Geometry check sheet. Reference: drawing and pictorial views, mm from the part's lowest x, y, z. Coordinates: 2 decimals unless noted, no trailing zeros. Write each loop counter-clockwise with the first axis right and the second up, starting at its lowest first coordinate (ties: lowest second). Pieces come first, ordered by that corner, then holes. Notation, with made-up numbers: (16, -30.5) -> (68, -30.5) arc R32 ccw to (68, 6.5) -> close; hole circle Ø11 at (89.25, -22.75). An arc over 180 degrees is marked (long way). Use a Markdown table: item, result.
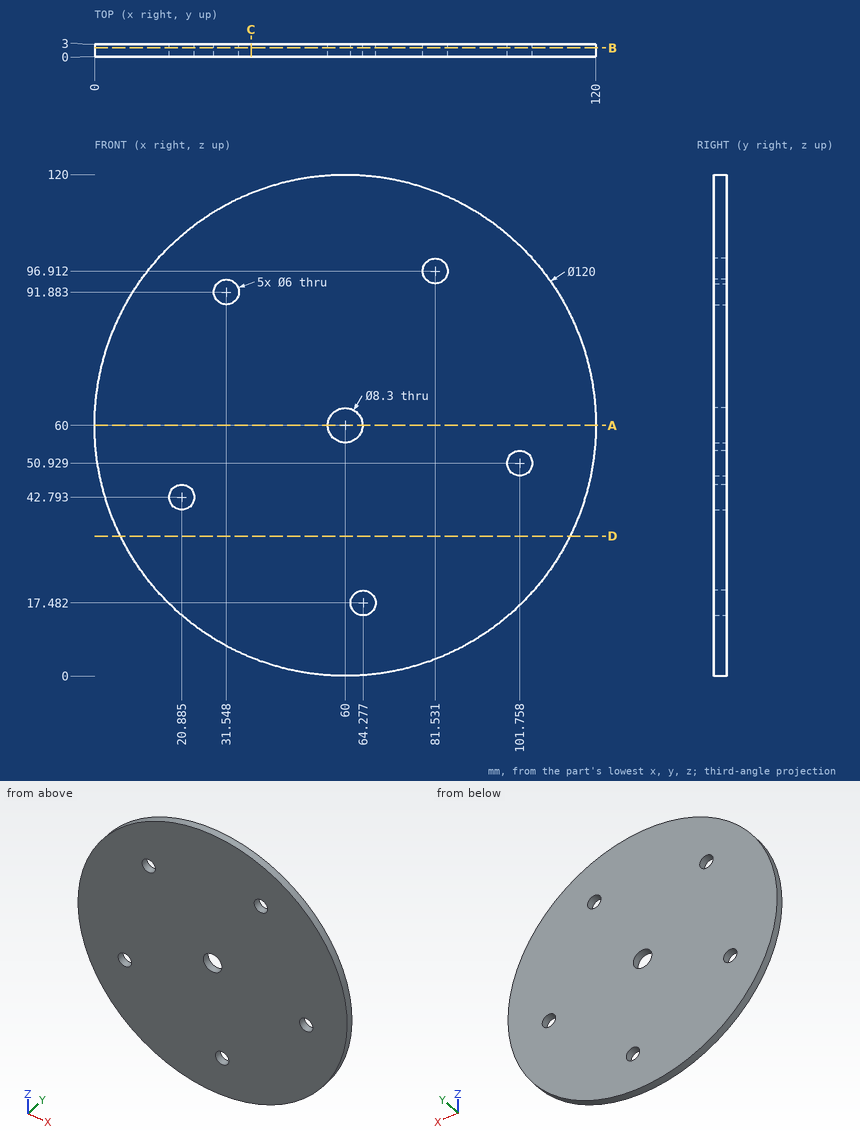
Item 1: Section check D-D on z = 33.5. Record the boundary of the cut face in (x, y), then the cut area to 3 significant figures.
Answer block:
| item | result |
|---|---|
| outline | (6.17, 0) -> (113.83, 0) -> (113.83, 3) -> (6.17, 3) -> close |
| area | 323 mm^2 |
Item 2: Section check B-B on y = 2.1. Count the separate pieces of the cut face and the enclosed holes in it, then the cut area to 3 significant figures.
Answer block:
| item | result |
|---|---|
| separate pieces | 1 |
| enclosed holes | 6 |
| area | 11,100 mm^2 |
Item 3: Section check A-A on z = 60. Record the boundary of the cut face in (x, y).
Answer block:
| item | result |
|---|---|
| outline | (0, 0) -> (55.85, 0) -> (55.85, 3) -> (0, 3) -> close; (64.15, 0) -> (120, 0) -> (120, 3) -> (64.15, 3) -> close |
Item 4: Thickness scan on L1, parallel to X at y = 1, z = 95 (1 decimal); L2, parallel to X at y = 2.85, z = 45.5 (1 decimal); L3, parallel to Z at x = 103.5, y = 0.65 (1 decimal). Record the ranges inside material, lowest first. Write a range as [from, to].
Answer block:
| item | result |
|---|---|
| L1 | x = [11.3, 79.2], [83.8, 108.7] |
| L2 | x = [1.8, 19.6], [22.2, 118.2] |
| L3 | z = [18.7, 48.5], [53.4, 101.3] |
Item 5: Depth check by flat-ended pin: P1, Ø1.5, axis at x = 13.5, y = 0.5, coming from the -Z side. Enter the tip coordinate at first touch or a pass-through.
Answer block:
| item | result |
|---|---|
| P1 | stops at z = 21.18 |
Item 6: Section check C-C on x = 37.5. Record the boundary of the cut face in (y, z), then the cut area to 3 significant figures.
Answer block:
| item | result |
|---|---|
| outline | (0, 4.38) -> (3, 4.38) -> (3, 115.62) -> (0, 115.62) -> close |
| area | 334 mm^2 |
